Part model, mm, in its own coordinate system. Face numbers are marked on the shaded views. Coordinates: 2 decimals unless noted, no trailing zeros. Order: outer loops, then holes, each group sorted by start corner. A loop starts at its lowest first (then second) coordinate and runs counter-clockwise, first axis right, second up.
1) Cut at A-A (y = -1.25). List the corners of the cut face in (x, z).
2) Pin check, flat tips, straight feed: pin 1 Ø4.5 at (x, z) = (-105, -90) entering from +Y; pin 2 Ø4 at (x, z) = (103.7, -88.7) entering from +Y. Stop position of each tip, or through.
3) Cut at B-B (x = 70). List the corners of the cut face in (y, z), and give its area (4 significant figures).
4) Wall check: L1, parallel to Z at x = -103.7, y = -0.85; L2, parallel to Z at x = 103.7, y = 3.1; L3, parallel to X at y = -1.15, z = -88.7. Give the ranges that are in metal, low to high.
5) Cut at C-C (z = 2). List the corners of the cut face in (x, y).
6) Mould opens along X. For the marked faces 1 and 2 say: +X half, -X half, draft (parallel to the pull), parting line (faces both ways), or undercut.
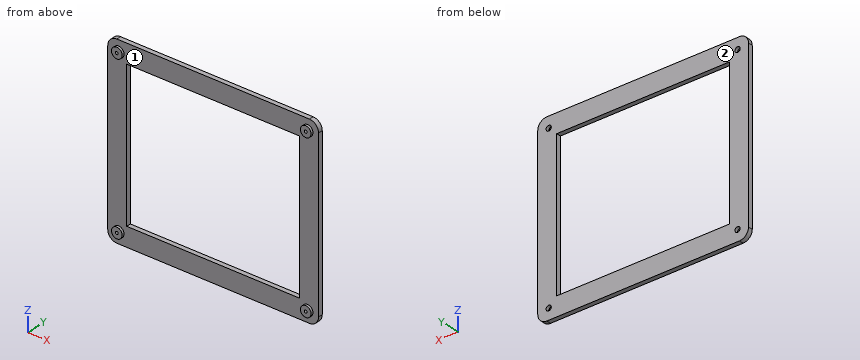
```python
from build123d import *

# Parameters (mm, degrees)
SKETCH1_W               = 231.4
SKETCH1_H               = 201.4
SKETCH1_W_2             = 189.9
SKETCH1_H_2             = 159.9
BOSS_EXTRUDE1_DEPTH     = 5
FILLET1_R               = 10
SKETCH2_R               = 5.85
BOSS_EXTRUDE2_DEPTH     = 2.5
SKETCH3_R               = 1.55
CUT_EXTRUDE1_DEPTH      = 7.5
SKETCH4_R               = 2.85
CUT_EXTRUDE2_DEPTH      = 3.5
MIRROR4_COPY_1_SKETCH_R = 5.85
MIRROR4_COPY_1_DEPTH    = 2.5
MIRROR4_COPY_2_SKETCH_R = 1.55
MIRROR4_COPY_2_DEPTH    = 7.5
MIRROR4_COPY_3_SKETCH_R = 2.85
MIRROR4_COPY_3_DEPTH    = 3.5


with BuildPart() as part:
    # Sketch1 → Boss-Extrude1 (new body)
    with BuildSketch(Plane(origin=(0, 0, 0), x_dir=(1, 0, 0), z_dir=(0, 1, 0))):
        Rectangle(SKETCH1_W, SKETCH1_H)
        Rectangle(SKETCH1_W_2, SKETCH1_H_2, mode=Mode.SUBTRACT)
    extrude(amount=BOSS_EXTRUDE1_DEPTH)

    # Fillet1
    fillet1_edges = [part.edges().sort_by_distance(p)[0] for p in [
        (-115.7, 2.5, -100.7),
        (115.7, 2.5, -100.7),
        (115.7, 2.5, 100.7),
        (-115.7, 2.5, 100.7),
    ]]
    fillet(fillet1_edges, radius=FILLET1_R)

    # Sketch2 → Boss-Extrude2 (add)
    with BuildSketch(Plane.XZ):
        with Locations((-103.7, 88.7)):
            Circle(SKETCH2_R)
    boss_extrude2 = extrude(amount=BOSS_EXTRUDE2_DEPTH)

    # Sketch3 → Cut-Extrude1 (cut)
    with BuildSketch(Plane(origin=(0, 5, 0), x_dir=(1, 0, 0), z_dir=(0, 1, 0))):
        with Locations((-103.7, -88.7)):
            Circle(SKETCH3_R)
    cut_extrude1 = extrude(amount=-CUT_EXTRUDE1_DEPTH, mode=Mode.SUBTRACT)

    # Sketch4 → Cut-Extrude2 (cut)
    with BuildSketch(Plane(origin=(0, 5, 0), x_dir=(1, 0, 0), z_dir=(0, 1, 0))):
        with Locations((-103.7, -88.7)):
            Circle(SKETCH4_R)
    cut_extrude2 = extrude(amount=-CUT_EXTRUDE2_DEPTH, mode=Mode.SUBTRACT)

    # Mirror3: Boss-Extrude2, Cut-Extrude1, Cut-Extrude2 across plane
    add(boss_extrude2.mirror(Plane(origin=(0, 0, 0), x_dir=(0, 0, 1), z_dir=(1, 0, 0))))
    add(cut_extrude1.mirror(Plane(origin=(0, 0, 0), x_dir=(0, 0, 1), z_dir=(1, 0, 0))), mode=Mode.SUBTRACT)
    add(cut_extrude2.mirror(Plane(origin=(0, 0, 0), x_dir=(0, 0, 1), z_dir=(1, 0, 0))), mode=Mode.SUBTRACT)

    # Mirror4: Boss-Extrude2, Cut-Extrude1, Cut-Extrude2 across plane
    add(boss_extrude2.mirror(Plane.XY))
    add(cut_extrude1.mirror(Plane.XY), mode=Mode.SUBTRACT)
    add(cut_extrude2.mirror(Plane.XY), mode=Mode.SUBTRACT)

    # Mirror4 copy 1 sketch → Mirror4 copy 1 (add)
    with BuildSketch(Plane(origin=(0, 0, 0), x_dir=(-1, 0, 0), z_dir=(0, -1, 0))):
        with Locations((-103.7, 88.7)):
            Circle(MIRROR4_COPY_1_SKETCH_R)
    extrude(amount=MIRROR4_COPY_1_DEPTH)

    # Mirror4 copy 2 sketch → Mirror4 copy 2 (cut)
    with BuildSketch(Plane(origin=(0, 5, 0), x_dir=(-1, 0, 0), z_dir=(0, 1, 0))):
        with Locations((-103.7, -88.7)):
            Circle(MIRROR4_COPY_2_SKETCH_R)
    extrude(amount=-MIRROR4_COPY_2_DEPTH, mode=Mode.SUBTRACT)

    # Mirror4 copy 3 sketch → Mirror4 copy 3 (cut)
    with BuildSketch(Plane(origin=(0, 5, 0), x_dir=(-1, 0, 0), z_dir=(0, 1, 0))):
        with Locations((-103.7, -88.7)):
            Circle(MIRROR4_COPY_3_SKETCH_R)
    extrude(amount=-MIRROR4_COPY_3_DEPTH, mode=Mode.SUBTRACT)


solid = part.part
```
Geometry check:
1. outline: circle Ø11.7 at (-103.7, -88.7); circle Ø11.7 at (-103.7, 88.7); circle Ø11.7 at (103.7, -88.7); circle Ø11.7 at (103.7, 88.7); hole circle Ø3.1 at (-103.7, -88.7); hole circle Ø3.1 at (-103.7, 88.7); hole circle Ø3.1 at (103.7, -88.7); hole circle Ø3.1 at (103.7, 88.7)
2. pin 1: stops at y = 5
2. pin 2: stops at y = 1.5
3. outline: (0, -100.7) - (5, -100.7) - (5, -79.95) - (0, -79.95) - close; (0, 79.95) - (5, 79.95) - (5, 100.7) - (0, 100.7) - close
3. area: 207.5 mm2
4. L1: z = -94.55 to -90.25, -87.15 to -82.85, 82.85 to 87.15, 90.25 to 94.55
4. L2: z = -100.7 to -91.55, -85.85 to 85.85, 91.55 to 100.7
4. L3: x = -109.55 to -105.25, -102.15 to -97.85, 97.85 to 102.15, 105.25 to 109.55
5. outline: (-115.7, 0) - (-94.95, 0) - (-94.95, 5) - (-115.7, 5) - close; (94.95, 0) - (115.7, 0) - (115.7, 5) - (94.95, 5) - close
6. face 1: undercut
6. face 2: draft
